CAD build for the part. Positions are in the model's coordinates, mm. Face numbers are marked on the shaded views. Round coordinates to 2 decimals unless told otherwise and drop trailing zeros. Write each loop counter-clockwise with the first axis right and the second up, starting at its lowest first coordinate (ties: lowest second). Pieces come first, ordered by that corner, then holes. Notation, with made-up numbers: (14, 89.25) - (38, 89.25) arc R24 ccw to (38, 117.25) - close; hole circle Ø1 at (-29, -20.75). An arc over 180 degrees is marked (long way). Put each result on its own line as item: value. Start each with the question number.
Item 1: Cut at C-C (z = 10.5). Give the cut face in (x, y) (3 decimals).
Item 2: Mould opens along Y. For the marked faces 1, 2, 3 and 4 say: released by +Y, released by -Y, zero draft, split by the parting line, or undercut.
Item 3: Cut at A-A (y = -11). Give the cut face in (x, z) (3 decimals).
Item 4: Cut at D-D (x = 34). Give the cut face in (y, z).
Item 5: Pin check, flat tip, straight feed: pin 1 Ø18.5 at (x, y) = (4.5, -13.5) entering from +Z. Stop position of the tip, or through.
Item 6: Cut at B-B (x = 47). Give the cut face in (y, z).
Item 7: Drill centre lines: line 1 (X direction, y = 0.5, z = 1); line 2 (Y direction, x = 29, z = 7.75); line 3 (X direction, y = -40.5, z = 11.75). Where is each one in solid material? Low to high. Write a range as from..to.
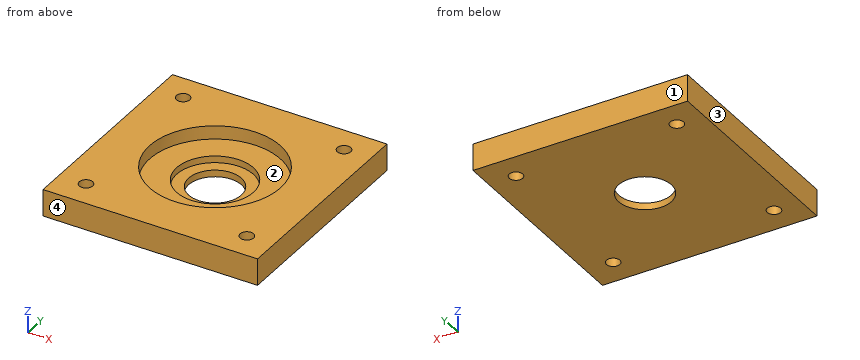
```python
from build123d import *

# Parameters (mm, degrees)
F0_R     = 3.175
F0_R_2   = 31.0007
F1_DEPTH = 12.7
F0_R_3   = 18.161
F2_DEPTH = 6.35
F0_R_4   = 12.4841
F3_DEPTH = 3.175


with BuildPart() as f1:
    # F0 (on Top) → F1 (new body)
    with BuildSketch(Plane.XY):
        Polygon((-41.051641, 50.779698), (-41.051641, 0), (-41.051641, -50.820302), (60.548359, -50.820302), (60.548359, 50.779698), align=None)
        with Locations((-28.351641, -38.120302)):
            Circle(F0_R, mode=Mode.SUBTRACT)
        with Locations((47.848359, -38.120302)):
            Circle(F0_R, mode=Mode.SUBTRACT)
        with Locations((9.748359, -0.020302)):
            Circle(F0_R_2, mode=Mode.SUBTRACT)
        with Locations((-28.351641, 38.079698)):
            Circle(F0_R, mode=Mode.SUBTRACT)
        with Locations((47.848359, 38.079698)):
            Circle(F0_R, mode=Mode.SUBTRACT)
    extrude(amount=F1_DEPTH)

    # F0 (on Top) → F2 (join)
    with BuildSketch(Plane.XY):
        with Locations((9.748359, -0.020302)):
            Circle(F0_R_2)
        with Locations((9.748359, -0.020302)):
            Circle(F0_R_3, mode=Mode.SUBTRACT)
    extrude(amount=F2_DEPTH)

    # F0 (on Top) → F3 (join)
    with BuildSketch(Plane.XY):
        with Locations((9.748359, -0.020302)):
            Circle(F0_R_3)
        with Locations((9.748359, -0.020302)):
            Circle(F0_R_4, mode=Mode.SUBTRACT)
    extrude(amount=F3_DEPTH)


solid = f1.part
```
Output values:
1. outline: (-41.052, -50.82) - (60.548, -50.82) - (60.548, 50.78) - (-41.052, 50.78) - close; hole circle Ø6.35 at (-28.352, -38.12); hole circle Ø6.35 at (-28.352, 38.08); hole circle Ø62.001 at (9.748, -0.02); hole circle Ø6.35 at (47.848, -38.12); hole circle Ø6.35 at (47.848, 38.08)
2. face 1: released by +Y
2. face 2: undercut
2. face 3: zero draft
2. face 4: released by -Y
3. outline: (-41.052, 0) - (3.807, 0) - (3.807, 3.175) - (-4.718, 3.175) - (-4.718, 6.35) - (-19.243, 6.35) - (-19.243, 12.7) - (-41.052, 12.7) - close; (15.69, 0) - (60.548, 0) - (60.548, 12.7) - (38.74, 12.7) - (38.74, 6.35) - (24.214, 6.35) - (24.214, 3.175) - (15.69, 3.175) - close
4. outline: (-50.82, 0) - (50.78, 0) - (50.78, 12.7) - (19.29, 12.7) - (19.29, 6.35) - (-19.33, 6.35) - (-19.33, 12.7) - (-50.82, 12.7) - close
5. pin 1: z = 6.35
6. outline: (-50.82, 0) - (-41.18, 0) - (-41.18, 12.7) - (-50.82, 12.7) - close; (-35.06, 0) - (35.02, 0) - (35.02, 12.7) - (-35.06, 12.7) - close; (41.14, 0) - (50.78, 0) - (50.78, 12.7) - (41.14, 12.7) - close
7. line 1: -41.05..-2.72, 22.22..60.55
7. line 2: -50.82..-24.32, 24.28..50.78
7. line 3: -41.05..-30.45, -26.25..45.75, 49.95..60.55
